```python
from build123d import *

# Parameters (mm, degrees)
PAD_DEPTH = 4
FILLET_R  = 1


with BuildPart() as part:
    # Sketch → Pad (new body)
    with BuildSketch(Plane.XY):
        Polygon((0, 0), (75, 0), (112.5, 37.5), (37.5, 37.5), align=None)
    extrude(amount=PAD_DEPTH)

    # Fillet
    fillet_edges = [part.edges().sort_by_distance(p)[0] for p in [
        (0, 0, 2),
        (75, 0, 2),
        (37.5, 0, 0),
        (37.5, 0, 4),
        (112.5, 37.5, 2),
        (93.75, 18.75, 0),
        (93.75, 18.75, 4),
        (37.5, 37.5, 2),
        (75, 37.5, 0),
        (75, 37.5, 4),
        (18.75, 18.75, 0),
        (18.75, 18.75, 4),
    ]]
    fillet(fillet_edges, radius=FILLET_R)


solid = part.part
```
Work out the finished part from the listing and answer in its coordinate system (mm). Round coordinates to 2 decimals unless told otherwise and drop trailing zeros. Loops run counter-clockwise (first coordinate to the right, second up) from the corner with the lowest first, then second, coordinate; pieces in that order, holes last.
(1) The part is cut by section A-A, the plane z = 2.2. Give the vertices of the cut face in (x, y), and give its area (3 significant figures).
Computed values:
outline: (1.71, 1.71) arc R1 ccw to (2.41, 0) - (74.59, 0) arc R1 ccw to (75.29, 0.29) - (110.79, 35.79) arc R1 ccw to (110.09, 37.5) - (37.91, 37.5) arc R1 ccw to (37.21, 37.21) - close
area: 2,810 mm2
(2) Each of these flat-tipped pins is pushed along its axis until it touches: P1, Ø12, axis at x = 89.5, y = 24.5, coming from the -Z side; P2, Ø2, axis at y = 23.5, z = 1.5, coming from the -X side. Where does it stop, or does it pass through?
Computed values:
P1: stops at z = 0
P2: stops at x = 22.5
(3) Find the intervals of material crossed by L1, parallel to X at y = 6.5, z = 2.2; L2, parallel to Y at x = 12, z = 0.75; L3, parallel to Y at x = 22.5, z = 0.25, in increasing order.
Computed values:
L1: x = 6.5 to 81.5
L2: y = 0.03 to 11.96
L3: y = 0.34 to 22.02
